The figure shows three views and two pictorial views of one solid part (mm, origin at its lowest corner). Answer the questions. A direction names the side the tool comes from. Coordinates: 2 decimals unless noted, no trailing zeros. Order: outer loops, then holes, each group sorted by start corner. A loop starts at its lowest first (then second) coordinate and runs counter-clockwise, first axis right, second up. Notation, with made-up numbers: (-14.5, 45) - (40.5, 45) arc R20 ccw to (40.5, 59) - close; hole circle Ø11 at (5, -14). An arc over 180 degrees is marked (long way). Use one line per item in the form item = value. Start each with the question number.
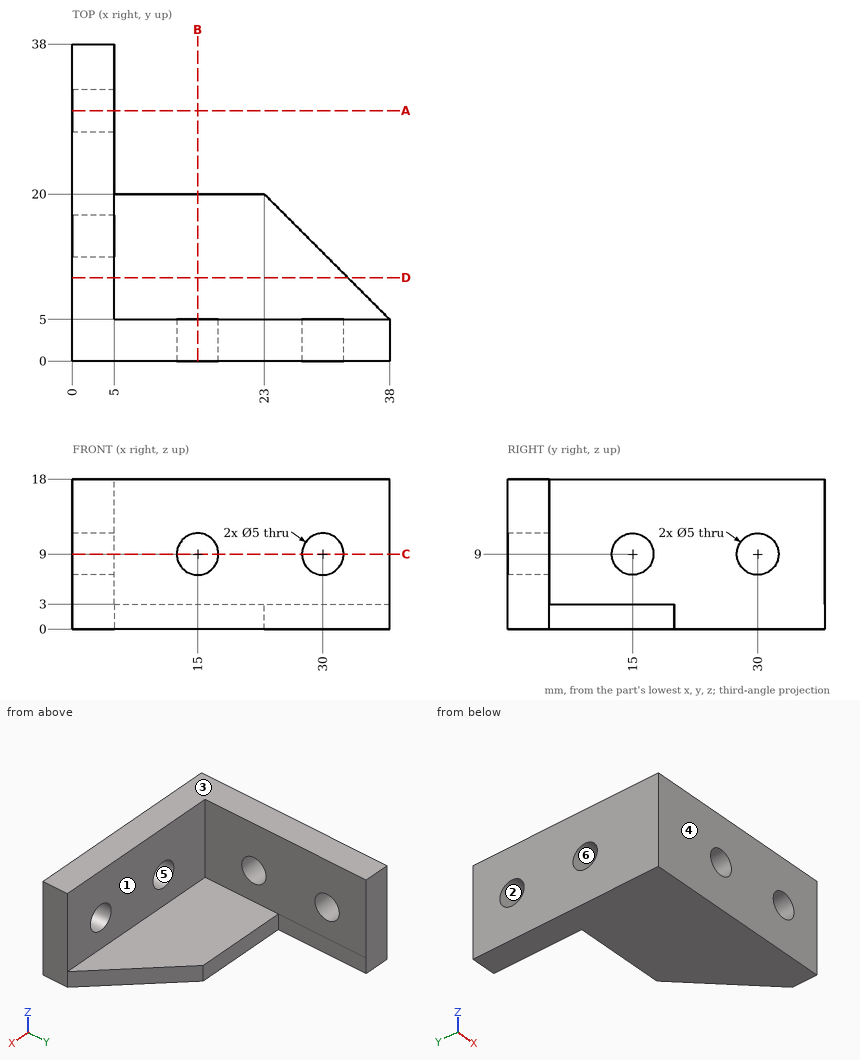
Q1. Which of the six approach directions +Z, -Z, +X, -X, +Y, -Y give full straight-line access (tool end or side, diameter ignored) to the marked faces 1 and 2?
Q2. A cutting plane is placed at B-B (x = 15). Give the vertices of the cut face in (y, z).
Q3. A cutting plane is placed at D-D (y = 10). Give the vertices of the cut face in (x, z), then the cut area to 3 significant figures.
Q4. A cutting plane is placed at C-C (z = 9). Give the vertices of the cut face in (x, y), then the cut area to 3 significant figures.
Q5. For a pull along Z with two mould halves and no side action, classify the marked faces 3, 4, 5 and 6 as +Z half, -Z half, draft (parallel to the pull), parting line (faces both ways), or undercut.
Q6. Consider probe 1 along Z at (x, y) = (3, 15); probe 2 along Y at (x, z) = (16, 16.75). Determine where each line is inside the solid, lowest interval first.
Q7. Given P1, Ø1.5, axis at x = 10, z = 1.5, coming from the +Y side; P2, Ø1, axis at y = 30, z = 14.5, coming from the +X side; P3, Ø6, axis at x = 10.5, y = 8.5, coming from the +Z side; P4, Ø4, axis at x = 15, z = 9, coming from the +Y side, each flat-ended and moving along its own axis, determine where each tip first touches the part or whether it passes through.
Q8. A cutting plane is placed at A-A (y = 30). Give the vertices of the cut face in (x, z).
Result sheet:
q1.face_1 = +Z, +X, +Y
q1.face_2 = +X, -X
q2.outline = (0, 0) - (20, 0) - (20, 3) - (5, 3) - (5, 6.5) - (0, 6.5) - close; (0, 11.5) - (5, 11.5) - (5, 18) - (0, 18) - close
q3.outline = (0, 0) - (33, 0) - (33, 3) - (5, 3) - (5, 18) - (0, 18) - close
q3.area = 174 mm^2
q4.outline = (0, 0) - (12.5, 0) - (12.5, 5) - (5, 5) - (5, 12.5) - (0, 12.5) - close; (0, 17.5) - (5, 17.5) - (5, 27.5) - (0, 27.5) - close; (0, 32.5) - (5, 32.5) - (5, 38) - (0, 38) - close; (17.5, 0) - (27.5, 0) - (27.5, 5) - (17.5, 5) - close; (32.5, 0) - (38, 0) - (38, 5) - (32.5, 5) - close
q4.area = 255 mm^2
q5.face_3 = +Z half
q5.face_4 = draft
q5.face_5 = undercut
q5.face_6 = undercut
q6.probe_1 = 0 to 6.5, 11.5 to 18
q6.probe_2 = 0 to 5
q7.P1 = 20
q7.P2 = 5
q7.P3 = 3
q7.P4 = through
q8.outline = (0, 0) - (5, 0) - (5, 6.5) - (0, 6.5) - close; (0, 11.5) - (5, 11.5) - (5, 18) - (0, 18) - close
